from build123d import *

# Parameters (mm, degrees)
F0_R     = 1.7272
F1_DEPTH = 6.35
F2_R     = 1.7272
F2_R_2   = 2.15265
F2_W     = 12.7
F2_H     = 71.12
F2_R_3   = 21.510772
F3_DEPTH = 6.35
F4_R     = 3.96875


with BuildPart() as f1:
    # F0 (on Top) → F1 (new body)
    with BuildSketch(Plane.XY):
        Polygon((88.9, 153.979317), (0, 177.8), (-1651, 177.8), (-1651, -177.8), (0, -177.8), (88.9, -153.979317), (153.979317, -88.9), (177.8, 0), (153.979317, 88.9), align=None)
        with Locations((-1621.63125, -72.23125)):
            Circle(F0_R, mode=Mode.SUBTRACT)
        with Locations((-1477.16875, -72.23125)):
            Circle(F0_R, mode=Mode.SUBTRACT)
        with Locations((-1621.63125, 72.23125)):
            Circle(F0_R, mode=Mode.SUBTRACT)
        with Locations((-1477.16875, 72.23125)):
            Circle(F0_R, mode=Mode.SUBTRACT)
    extrude(amount=F1_DEPTH)

    # F2 (on face) → F3 (cut, through all)
    with BuildSketch(Plane.XY.offset(6.35)):
        with Locations((-568.091641, -11.995942)):
            Circle(F2_R)
        with Locations((-599.841641, -11.995942)):
            Circle(F2_R)
        with Locations((-599.841641, 8.641558)):
            Circle(F2_R)
        with Locations((-568.091641, 8.641558)):
            Circle(F2_R)
        with Locations((-1028.355112, -1.491475)):
            Circle(F2_R)
        with Locations((-1028.355112, -22.128975)):
            Circle(F2_R)
        with Locations((-1060.105112, -22.128975)):
            Circle(F2_R)
        with Locations((-1060.105112, -1.491475)):
            Circle(F2_R)
        with Locations((-438.049884, 118.36762)):
            Circle(F2_R_2)
        with Locations((-507.785101, 118.367619)):
            Circle(F2_R_2)
        with Locations((-507.785101, -118.36762)):
            Circle(F2_R_2)
        with Locations((-438.049884, -118.36762)):
            Circle(F2_R_2)
        with Locations((-1169.146759, -131.855036)):
            Circle(F2_R_2)
        with Locations((-1120.411652, -131.855036)):
            Circle(F2_R_2)
        with Locations((-1169.146759, 104.880203)):
            Circle(F2_R_2)
        with Locations((-1120.411652, 104.880203)):
            Circle(F2_R_2)
        with Locations((-1290.943305, 71.12)):
            Rectangle(F2_W, F2_H)
        with Locations((-1290.943305, -71.12)):
            Rectangle(F2_W, F2_H)
        with Locations((-1337.209023, -10.512984)):
            Circle(F2_R_3)
        with Locations((-1242.325218, 10.627991)):
            Circle(F2_R_3)
    extrude(amount=-F3_DEPTH, mode=Mode.SUBTRACT)

    # F4
    f4_edges = [f1.edges().sort_by_distance(p)[0] for p in [
        (0, -177.8, 3.175),
        (88.9, -153.979317, 3.175),
        (153.979317, -88.9, 3.175),
        (177.8, 0, 3.175),
        (153.979317, 88.9, 3.175),
        (88.9, 153.979317, 3.175),
        (0, 177.8, 3.175),
        (-1651, 177.8, 3.175),
        (-1651, -177.8, 3.175),
    ]]
    fillet(f4_edges, radius=F4_R)


solid = f1.part
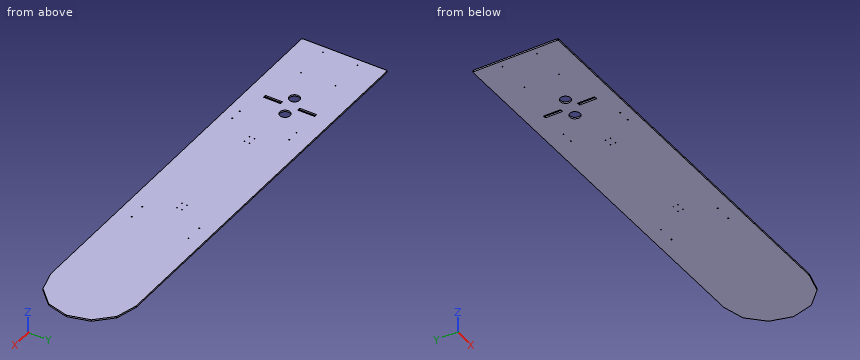
The model under review builds one solid part; all positions refer to its coordinate system, in mm. Coordinates: 2 decimals unless noted, no trailing zeros. Loops run counter-clockwise (first coordinate to the right, second up) from the corner with the lowest first, then second, coordinate; pieces in that order, holes last. Notation, with made-up numbers: M 6,5.25 L 52,5.25 A25 ccw 52,44.25 Z; hole C 73,-36 d10. An arc over 180 degrees is marked long. Put each result on its own line as item: value. Start each with the question number.
Q1. Add section A-A (x = -1242). Write out the cut boundary in (y, z).
Q2. Add section B-B (z = 2.75). Count the separate pieces of the cut face and the enclosed holes in it, and give its area (3 significant figures).
Q3. Clearance check with a flat-ended pin moving along its axis: pin 1 (5 mm diameter, centred on x = -438.05, y = 118.37, fed in from +Z). State where the tip first meets the part, or that it passes through.
Q4. Wall thickness on line 1 (X direction, y = 104, z = 5.25); line 2 (X direction, y = -73.5, z = 1.75); line 3 (X direction, y = -116.5, z = 2): over which ranges is each line inside the solid? List them lowest first.
Answers:
1. outline: M -177.8,0 L -10.88,0 L -10.88,6.35 L -177.8,6.35 Z; M 32.14,0 L 177.8,0 L 177.8,6.35 L 32.14,6.35 Z
2. separate pieces: 1
2. enclosed holes: 24
2. area: 630,000 mm^2
3. pin 1: stops at z = 6.35
4. line 1: x = -1651 to -1297.29, -1284.59 to -1171.11, -1167.18 to -1122.38, -1118.45 to 138.88
4. line 2: x = -1651 to -1622.8, -1620.46 to -1478.34, -1476 to -1297.29, -1284.59 to 158.11
4. line 3: x = -1651 to -508.86, -506.71 to -439.12, -436.98 to 126.38
